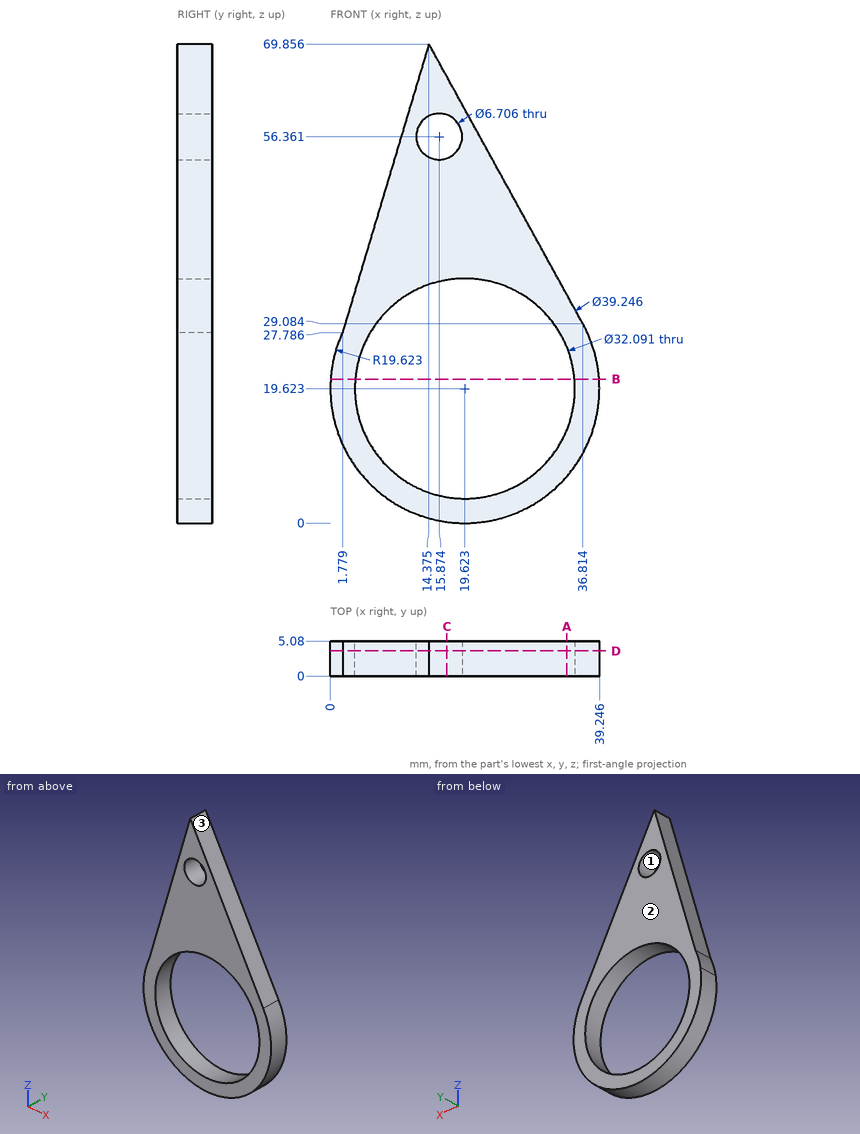
Could you check a few things on this drawing? It's one solid part, dimensions in mm from its lowest x, y, z. Round coordinates to 2 decimals unless told otherwise and drop trailing zeros. Order: outer loops, then holes, each group sorted by start corner. A loop starts at its lowest first (then second) coordinate and runs counter-clockwise, first axis right, second up.
(1) Imagine slicing it at B-B (z = 21). Write out the boundary of the cut face in (x, y).
Response values:
outline: (0.05, 0) - (3.64, 0) - (3.64, 5.08) - (0.05, 5.08) - close; (35.61, 0) - (39.2, 0) - (39.2, 5.08) - (35.61, 5.08) - close
(2) I'm going to push a flat-ended pin straight in: pin 1 (3 mm diameter, centred on x = 27.5, y = 4.5, fed in from -Z) (1 decimal). Where does the tip first touch, or does it pass through?
Response values:
pin 1: stops at z = 1.1
(3) Imagine slicing it at C-C (x = 17). Write out the boundary of the cut face in (y, z), plus the area to 3 significant figures.
Response values:
outline: (0, 0.18) - (5.08, 0.18) - (5.08, 3.79) - (0, 3.79) - close; (0, 35.45) - (5.08, 35.45) - (5.08, 53.2) - (0, 53.2) - close; (0, 59.52) - (5.08, 59.52) - (5.08, 65.09) - (0, 65.09) - close
area: 137 mm2
(4) Imagine slicing it at A-A (x = 34.5). Write out the boundary of the cut face in (y, z).
Response values:
outline: (0, 6.83) - (5.08, 6.83) - (5.08, 13.61) - (0, 13.61) - close; (0, 25.63) - (5.08, 25.63) - (5.08, 33.29) - (0, 33.29) - close
(5) Imagine slicing it at D-D (y = 3.65). Write out the boundary of the cut face in (x, z) (1 decimal).
Response values:
outline: (0.2, 22.6) arc R19.6 ccw (long way) to (36.8, 29.1) - (14.4, 69.9) - (1.8, 27.8) arc R19.6 ccw to start; hole circle Ø32.1 at (19.6, 19.6); hole circle Ø6.7 at (15.9, 56.4)
(6) If we mould it in two halves opening along X, with no side actions, what happens to the marked faces 1, 2 and 3? For each: released by +X, released by -X, zero draft, split by the parting line, or undercut.
Response values:
face 1: undercut
face 2: zero draft
face 3: released by +X
(7) Please list where these lines run through material, in increasing order: line 1 along X through (y, z) = (0.85, 27) (1 decimal); line 2 along X through (y, z) = (3.5, 30) (1 decimal); line 3 along Z through (x, y) = (33, 1.1) (1 decimal).
Response values:
line 1: x = 1.4 to 5.4, 33.9 to 37.8
line 2: x = 2.4 to 7.4, 31.9 to 36.3
line 3: z = 5.3 to 10.8, 28.5 to 36
